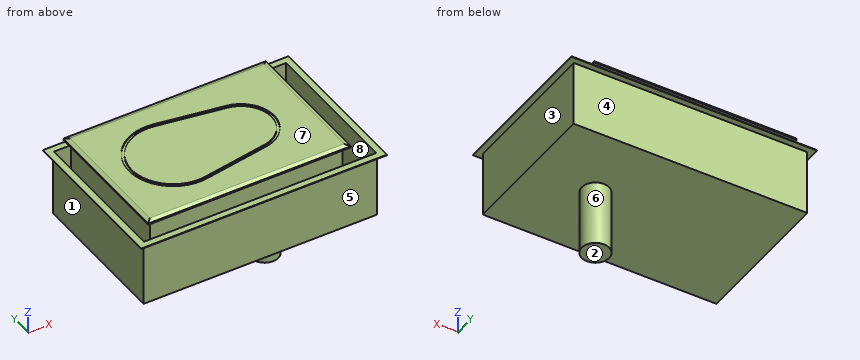
```python
from build123d import *

# Parameters (mm, degrees)
F0_W      = 466
F0_H      = 316
F1_DEPTH  = 6.35
F2_SIZE2  = 9.525
F2_SIZE   = 3.175
F4_DEPTH  = 2.54
F5_W      = 442
F5_H      = 295
F6_DEPTH  = 170
F7_R      = 31.5
F8_DEPTH  = 152.4
F10_START = -19.05
F9_W      = 537
F9_H      = 338
F10_DEPTH = 152.95
F11_T     = -1.524
F12_START = -19.05
F9_W_2    = 565
F9_H_2    = 366
F12_DEPTH = 1.524


with BuildPart() as f1:
    # F0 (on Top) → F1 (new body)
    with BuildSketch(Plane.XY):
        with Locations((-233, 158)):
            Rectangle(F0_W, F0_H)
    extrude(amount=F1_DEPTH)

    # F2
    f2_edges = [f1.edges().sort_by_distance(p)[0] for p in [
        (-233, 0, 6.35),
        (0, 158, 6.35),
        (-233, 316, 6.35),
        (-466, 158, 6.35),
    ]]
    chamfer(f2_edges, length=F2_SIZE, length2=F2_SIZE2)

    # F3 (on face) → F4 (cut)
    with BuildSketch(Plane.XY.offset(6.35)):
        with BuildLine():
            Line((-142.5426133743, 233.1967378452), (-294.5301511658, 258.258317127))
            ThreePointArc((-294.5301511658, 258.258317127), (-412.66, 158.012), (-294.5301511658, 57.765682873))
            Line((-294.5301511658, 57.765682873), (-142.5426133743, 82.8272621548))
            ThreePointArc((-142.5426133743, 82.8272621548), (-78.74, 158.012), (-142.5426133743, 233.1967378452))
        make_face()
        with BuildLine():
            Line((-143.5757292344, 89.0926588426), (-295.5632670258, 64.0310795608))
            ThreePointArc((-295.5632670258, 64.0310795608), (-406.3099981074, 158.012), (-295.5632670258, 251.9929204392))
            Line((-295.5632670258, 251.9929204392), (-143.5757292344, 226.9313411574))
            ThreePointArc((-143.5757292344, 226.9313411574), (-85.0900018926, 158.012), (-143.5757292344, 89.0926588426))
        make_face(mode=Mode.SUBTRACT)
    extrude(amount=-F4_DEPTH, mode=Mode.SUBTRACT)

    # F5 (on Top) → F6 (join)
    with BuildSketch(Plane.XY):
        with Locations((-233, 159.5)):
            Rectangle(F5_W, F5_H)
    extrude(amount=-F6_DEPTH)

    # F7 (on face) → F8 (join)
    with BuildSketch(Plane(origin=(0, 0, -170), x_dir=(1, 0, 0), z_dir=(0, 0, -1))):
        with Locations((-103.5423949361, -153.4942388535)):
            Circle(F7_R)
    extrude(amount=F8_DEPTH)



with BuildPart() as f10:
    # F9 (on Top) → F10 (new body)
    with BuildSketch(Plane.XY.offset(F10_START)):
        with Locations((-221.5, 147)):
            Rectangle(F9_W, F9_H)
    extrude(amount=-F10_DEPTH)

    # F11
    f11_openings = [f10.faces().sort_by_distance(p)[0] for p in [
        (-221.5, 147, -19.05),
    ]]
    offset(amount=F11_T, openings=f11_openings)


with BuildPart() as f1_1:
    add(f1.part)

    add(f10.part)  # F12 merges F10
    # F9 (on Top) → F12 (join)
    with BuildSketch(Plane.XY.offset(F12_START)):
        with Locations((-221.5, 147)):
            Rectangle(F9_W_2, F9_H_2)
        with Locations((-221.5, 147)):
            Rectangle(F9_W, F9_H, mode=Mode.SUBTRACT)
    extrude(amount=-F12_DEPTH)


solid = f1_1.part
```
Part model, mm, in its own coordinate system. Face numbers are marked on the shaded views. A direction names the side the tool comes from. Coordinates: 2 decimals unless noted, no trailing zeros. Write each loop counter-clockwise with the first axis right and the second up, starting at its lowest first coordinate (ties: lowest second). Pieces come first, ordered by that corner, then holes.
Item 1: Probe line 1 (X direction, y = 222, z = -31.5); line 2 (Y direction, x = -407.5, z = -139.5); line 3 (Y direction, x = 14, z = -109). List the from-to ranges inside material, lowest first.
Item 2: Slice it at D-D (z = -287). Write the cut outline in (x, y), and give its area (3 significant figures).
Item 3: Mould opens along Y. For the marked faces 5, 6, 7 and 8 say: released by +Y, released by -Y, zero draft, split by the parting line, or undercut.
Item 4: Pin check, flat tips, straight feed: pin 1 (10 mm diameter, centred on x = -198, y = 89, fed in from -Z); pin 2 (3 mm diameter, centred on y = 101.5, z = -78.5, fed in from +X); pin 3 (1 mm diameter, centred on x = -119.5, z = 2, fed in from -Y). Stop position of each tip, or through.
Item 5: Slice it at A-A (z = -162). Write the cut outline in (x, y), and give its area (3 significant figures).
Item 6: Which spindle directions (+Z, -Z, +X, -X, +Y, -Y) get a long thin tool onto all of the face, cutting with end or side? Do the marked faces 1, 2, 3 and 4. Say none if no direction does.
Results found:
1. line 1: x = -490 to -488.48, -454 to -12, 45.48 to 47
1. line 2: y = -22 to -20.48, 12 to 307, 314.48 to 316
1. line 3: y = -22 to -20.48, 314.48 to 316
2. outline: circle Ø63 at (-103.54, 153.49)
2. area: 3,120 mm2
3. face 5: released by -Y
3. face 6: split by the parting line
3. face 7: zero draft
3. face 8: undercut
4. pin 1: stops at z = -172
4. pin 2: stops at x = 47
4. pin 3: stops at y = 0
5. outline: (-490, -22) - (47, -22) - (47, 316) - (-490, 316) - close; (-454, 12) - (-12, 12) - (-12, 307) - (-454, 307) - close; hole (-488.48, -20.48) - (45.48, -20.48) - (45.48, 314.48) - (-488.48, 314.48) - close
5. area: 133,000 mm2
6. face 1: -Z, -X, +Y, -Y
6. face 2: -Z, +X, -X, +Y, -Y
6. face 3: -Z, +X, +Y, -Y
6. face 4: -Z, +X, -X, +Y
